Source: three-view drawing plus pictorial views. Frame: mm from the lowest corner of the part. Give positions to 0.01 mm unless a question says otherwise; leave off trailing zeros. Loops run counter-clockwise (first coordinate to the right, second up) from the corner with the lowest first, then second, coordinate; pieces in that order, holes last. Notation, with made-up numbers: (45, 62.25) - (64, 62.25) arc R25 ccw to (64, 101.25) - close; hole circle Ø1 at (15.5, 43). An arc over 180 degrees is marked (long way). Put each result on its own line as item: value.
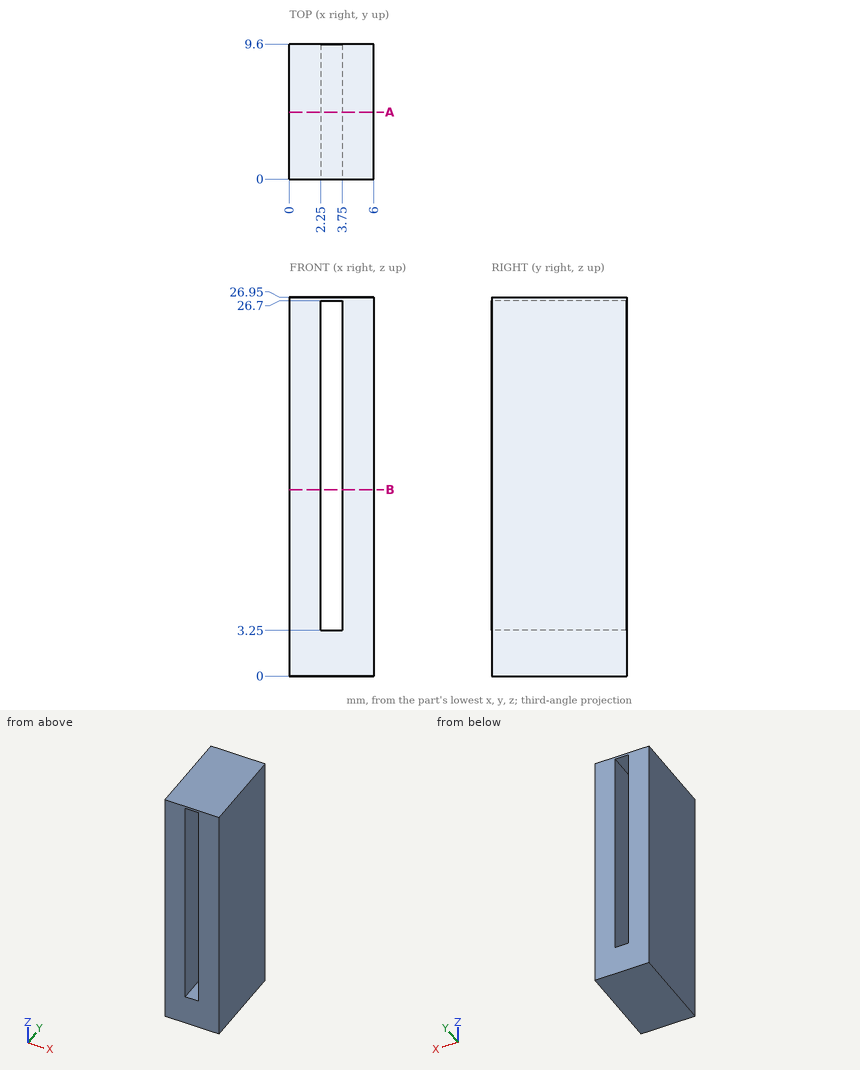
1) Section query A-A, the plane y = 4.75. Output: boundary loops of the cut face in (x, z), plus the area to 3 significant figures.
Check result:
outline: (0, 0) - (6, 0) - (6, 26.95) - (0, 26.95) - close; hole (2.25, 3.25) - (3.75, 3.25) - (3.75, 26.7) - (2.25, 26.7) - close
area: 127 mm²
2) Section query B-B, the plane z = 13.25. Output: boundary loops of the cut face in (x, y).
Check result:
outline: (0, 0) - (2.25, 0) - (2.25, 9.6) - (0, 9.6) - close; (3.75, 0) - (6, 0) - (6, 9.6) - (3.75, 9.6) - close
3) Material intervals for line 1 along Z through (x, y) = (2.9, 7); line 2 along X through (y, z) = (2, 3.75), sorted ascending. Write a range as [from, to].
Check result:
line 1: [0, 3.25], [26.7, 26.95]
line 2: [0, 2.25], [3.75, 6]
